Design review of the part shown in the three views and the two pictorial views. Dimensions are in mm from the part's minimum x, y and z. Give positions to 0.01 mm unless a question says otherwise; leave off trailing zeros. Loops run counter-clockwise (first coordinate to the right, second up) from the corner with the lowest first, then second, coordinate; pieces in that order, holes last. Notation, with made-up numbers: (62.25, -39) -> (114.25, -39) arc R22 cw to (114.25, -6) -> close; hole circle Ø9 at (22.25, 66). An arc over 180 degrees is marked (long way). Use CSV: the item, a comma, the result in double quotes. Start each with the question number.
Item 1: Wall thickness on line 1 along Z through (x, y) = (66.5, 7.75); line 2 along Z through (x, y) = (28.5, 16.75): over which ranges is each line inside the solid? List them lowest first. Write a range as from..to.
Item 2: We need section B-B (z = 1.75). State the section outline as (x, y) points, plus the area to 4 significant figures.
Item 3: We need section A-A (x = 48). State the section outline as (y, z) points, plus the area to 3 significant figures.
Item 4: We need section C-C (y = 14.25). State the section outline as (x, z) points.
Item 5: Clearance check with flat-ended pins moving along their axes: pin 1 (5 mm diameter, centred on x = 43, y = 8.5, fed in from +Z); pin 2 (1.5 mm diameter, centred on x = 62.5, y = 13.5, fed in from +Z); pin 3 (6 mm diameter, centred on x = 48.5, y = 7, fed in from +Z). State where each tip first meets the part, or that it passes through.
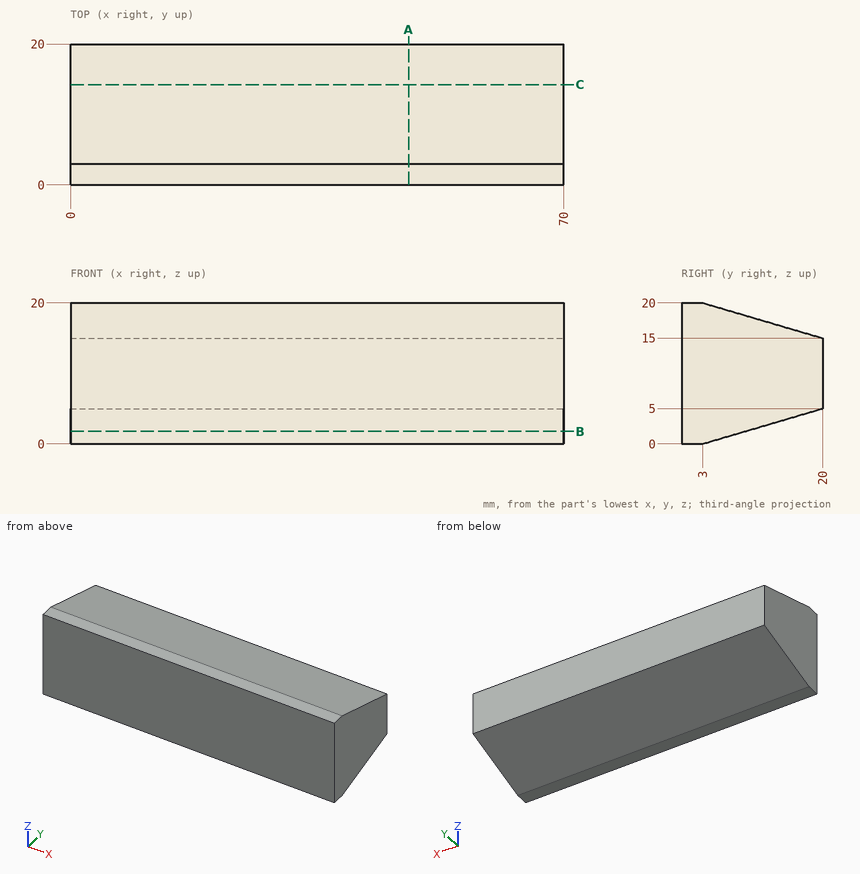
Results found:
1,line 1,"1.4..18.6"
1,line 2,"4.04..15.96"
2,outline,"(0, 0) -> (70, 0) -> (70, 8.95) -> (0, 8.95) -> close"
2,area,"626.5 mm²"
3,outline,"(0, 0) -> (3, 0) -> (20, 5) -> (20, 15) -> (3, 20) -> (0, 20) -> close"
3,area,"315 mm²"
4,outline,"(0, 3.31) -> (70, 3.31) -> (70, 16.69) -> (0, 16.69) -> close"
5,pin 1,"z = 19.12"
5,pin 2,"z = 17.13"
5,pin 3,"z = 19.71"
